Check sheet for the modelled part. Datum: model origin and axes. Units: mm. Give positions to 0.01 mm unless a question says otherwise; leave off trailing zeros. Order: outer loops, then holes, each group sorted by start corner. A loop starts at its lowest first (then second) coordinate and runs counter-clockwise, first axis right, second up. Notation, with made-up numbers: (-32, 15) -> (24, 15) arc R27 cw to (24, 40) -> close; hole circle Ø1 at (4, -28.75). An arc over 180 degrees is marked (long way). Answer in a Markdown table with one row per item. Add a question column.
(1) Cross-section at D-D (y = 27). Record the cut outline in (x, z), then the cut area to 3 significant figures.
(2) Cross-section at A-A (y = 16.5). Record the cut outline in (x, z), then the cut area to 3 significant figures.
(3) Thickness scan on L1, parallel to X at y = -6, z = 25; L2, parallel to Z at x = -10, y = 36.5; L3, parallel to Z at x = -19.5, y = -3. Record the ranges inside material, lowest first. Write a range as [from, to].
(4) Cross-section at B-B (x = -21). Record the cut outline in (y, z), then the cut area to 3 significant figures.
(5) Cross-section at C-C (z = 126.5). Record the cut outline in (x, y).
(6) Go/stop test with flat-tipped pins: pin 1 (3 mm diameter, centred on x = -7, z = 38, fed in from +Y); pin 2 (3 mm diameter, centred on y = 16.5, z = 133, fed in from -X); pin 3 (8 mm diameter, centred on x = 18, y = -8.5, fed in from +Z). Record where each tip stops, or that it passes through.
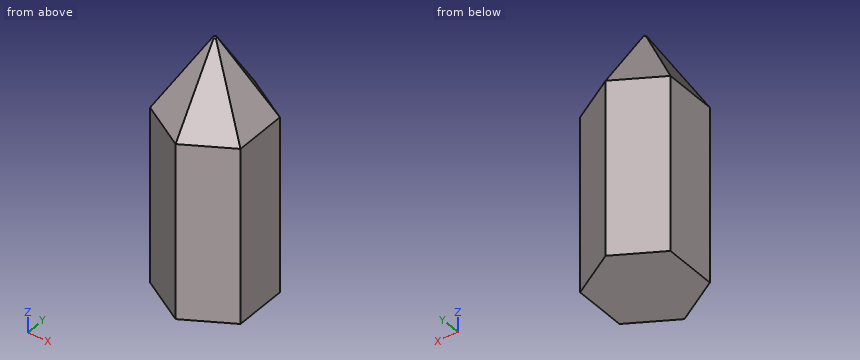
```python
from build123d import *

# Parameters (mm, degrees)
F1_DEPTH = 150
F2_SIZE2 = 25.9807621135
F2_SIZE  = 45


with BuildPart() as f1:
    # F0 (on Top) → F1 (new body)
    with BuildSketch(Plane.XY):
        Polygon((-15.4086170788, 13.843306002), (-24.4086170788, 29.4317632701), (-24.4086170788, -1.7451512661), align=None)
        Polygon((2.5913829212, 45.0202205382), (-24.4086170788, 29.4317632701), (-6.4086170788, 29.4317632701), align=None)
        Polygon((-6.4086170788, 29.4317632701), (-24.4086170788, 29.4317632701), (-15.4086170788, 13.843306002), align=None)
        Polygon((29.5913829212, 29.4317632701), (2.5913829212, 45.0202205382), (11.5913829212, 29.4317632701), align=None)
        Polygon((11.5913829212, 29.4317632701), (2.5913829212, 45.0202205382), (-6.4086170788, 29.4317632701), align=None)
        Polygon((-6.4086170788, -1.7451512661), (-24.4086170788, -1.7451512661), (2.5913829212, -17.3336085342), align=None)
        Polygon((-15.4086170788, 13.843306002), (-24.4086170788, -1.7451512661), (-6.4086170788, -1.7451512661), align=None)
        Polygon((20.5913829212, 13.843306002), (29.5913829212, 29.4317632701), (11.5913829212, 29.4317632701), align=None)
        Polygon((29.5913829212, -1.7451512661), (29.5913829212, 29.4317632701), (20.5913829212, 13.843306002), align=None)
        Polygon((11.5913829212, -1.7451512661), (2.5913829212, -17.3336085342), (29.5913829212, -1.7451512661), align=None)
        Polygon((-6.4086170788, -1.7451512661), (2.5913829212, -17.3336085342), (11.5913829212, -1.7451512661), align=None)
        Polygon((11.5913829212, -1.7451512661), (29.5913829212, -1.7451512661), (20.5913829212, 13.843306002), align=None)
        Polygon((11.5913829212, 29.4317632701), (-6.4086170788, 29.4317632701), (-15.4086170788, 13.843306002), (-6.4086170788, -1.7451512661), (11.5913829212, -1.7451512661), (20.5913829212, 13.843306002), align=None)
    extrude(amount=F1_DEPTH)

    # F2
    f2_edges = [f1.edges().sort_by_distance(p)[0] for p in [
        (16.091383, -9.53938, 150),
        (29.591383, 13.843306, 150),
        (16.091383, 37.225992, 150),
        (-10.908617, 37.225992, 150),
        (-24.408617, 13.843306, 150),
        (-10.908617, -9.53938, 150),
    ]]
    chamfer(f2_edges, length=F2_SIZE, length2=F2_SIZE2)


solid = f1.part
```
Answer below:
| question | item | result |
|---|---|---|
| 1 | outline | (-24.41, 0) -> (29.59, 0) -> (29.59, 105) -> (25.38, 112.3) -> (2.59, 132.03) -> (-20.2, 112.3) -> (-24.41, 105) -> close |
| 1 | area | 6,480 mm² |
| 2 | outline | (-24.41, 0) -> (29.59, 0) -> (29.59, 105) -> (7.19, 143.8) -> (2.59, 147.78) -> (-2.01, 143.8) -> (-24.41, 105) -> close |
| 2 | area | 6,910 mm² |
| 3 | L1 | x = [-17.04, 22.22] |
| 3 | L2 | z = [0, 106.88] |
| 3 | L3 | z = [0, 107.37] |
| 4 | outline | (-3.71, 0) -> (31.4, 0) -> (31.4, 105) -> (27.46, 110.9) -> (0.22, 110.9) -> (-3.71, 105) -> close |
| 4 | area | 3,870 mm² |
| 5 | outline | (-12, 5.42) -> (2.59, -3) -> (17.18, 5.42) -> (17.18, 22.27) -> (2.59, 30.69) -> (-12, 22.27) -> close |
| 6 | pin 1 | stops at y = 40.35 |
| 6 | pin 2 | stops at x = -9.11 |
| 6 | pin 3 | stops at z = 111.83 |
